Check sheet for the modelled part. Datum: model origin and axes. Units: mm. A direction names the side the tool comes from. Give positions to 0.01 mm unless a question says otherwise; leave off trailing zeros. Loops run counter-clockwise (first coordinate to the right, second up) from the corner with the lowest first, then second, coordinate; pieces in that order, holes last. Notation, with made-up numbers: (62.25, 86.5) - (105.25, 86.5) arc R10 ccw to (105.25, 94.5) - close; hole circle Ø7 at (-36.5, 26). An arc over 180 degrees is marked (long way). Use CSV: the item, a comma, the result in double quotes.
from build123d import *

# Parameters (mm, degrees)
SKETCH1_R               = 46.5
SKETCH1_R_2             = 36
BOSS_EXTRUDE1_DEPTH     = 2.325
BOSS_EXTRUDE2_START     = -2
SKETCH2_R               = 36
SKETCH2_R_2             = 33.63888889
BOSS_EXTRUDE2_DEPTH     = 2
CUT_EXTRUDE1_DEPTH      = 66.925127986
CUT_EXTRUDE1_DEPTH_BACK = 66.925127986
SKETCH3_R               = 1.25


with BuildPart() as part:
    # Sketch1 → Boss-Extrude1 (new, symmetric)
    with BuildSketch(Plane.XY):
        Circle(SKETCH1_R)
        Circle(SKETCH1_R_2, mode=Mode.SUBTRACT)
    extrude(amount=BOSS_EXTRUDE1_DEPTH, both=True)

    # Sketch2 → Boss-Extrude2 (add)
    with BuildSketch(Plane.XY.offset(2.325).offset(BOSS_EXTRUDE2_START)):
        Circle(SKETCH2_R)
        Circle(SKETCH2_R_2, mode=Mode.SUBTRACT)
    extrude(amount=BOSS_EXTRUDE2_DEPTH)

    # Sketch3 → Cut-Extrude1 (cut, two sides: drawn at the far end of the back side and taken through both)
    with BuildSketch(Plane.XY.offset(2.325).offset(-CUT_EXTRUDE1_DEPTH_BACK)):
        with Locations((-15.560126668, -38.202682603)):
            Circle(SKETCH3_R)
        with Locations((-32.576806282, -25.304430293)):
            Circle(SKETCH3_R)
        with Locations((-40.864556961, -5.625876321)):
            Circle(SKETCH3_R)
        with Locations((-38.202682603, 15.560126668)):
            Circle(SKETCH3_R)
        with Locations((-25.304430293, 32.576806282)):
            Circle(SKETCH3_R)
        with Locations((-5.625876321, 40.864556961)):
            Circle(SKETCH3_R)
        with Locations((15.560126668, 38.202682603)):
            Circle(SKETCH3_R)
        with Locations((32.576806282, 25.304430293)):
            Circle(SKETCH3_R)
        with Locations((40.864556961, 5.625876321)):
            Circle(SKETCH3_R)
        with Locations((38.202682603, -15.560126668)):
            Circle(SKETCH3_R)
        with Locations((25.304430293, -32.576806282)):
            Circle(SKETCH3_R)
        with Locations((5.625876321, -40.864556961)):
            Circle(SKETCH3_R)
    extrude(amount=CUT_EXTRUDE1_DEPTH + CUT_EXTRUDE1_DEPTH_BACK, mode=Mode.SUBTRACT)


solid = part.part
1. Scan lines: line 1 along Y through (x, z) = (14.5, -1.45); line 2 along Y through (x, z) = (16, 1.8); line 3 along X through (y, z) = (15.5, 0.6). Record each from-to range of solid material in increasing order.
Completed:
line 1,"y = -44.18 to -32.95, 32.95 to 37.54, 38.86 to 44.18"
line 2,"y = -43.66 to -29.59, 29.59 to 37.03, 39.37 to 43.66"
line 3,"x = -43.84 to -39.45, -36.95 to -29.86, 29.86 to 43.84"
2. Go/stop test with flat-tipped pins: pin 1 Ø3 at (x, y) = (25.3, -32.58) entering from -Z (3 decimals); pin 2 Ø1.5 at (x, y) = (-25.3, 32.58) entering from -Z; pin 3 Ø2 at (y, z) = (18, -1) entering from -X; pin 4 Ø2 at (y, z) = (29.5, -0.5) entering from -X. Record where each tip stops, or that it passes through.
Completed:
pin 1,"stops at z = -2.325"
pin 2,"passes through"
pin 3,"stops at x = -43.28"
pin 4,"stops at x = -36.74"
3. Set-up check for faces 5 (the face through (-39.124, 16.405, -0.033)), 6 (the face through (-30, 16, 0.325)): record each of +Z, -Z, +X, -X, +Y, -Y from which the full face is reachable in a straight line by a thin tool's end or side.
Completed:
face 5,"+Z, -Z"
face 6,"-Z"
4. Sectioned sample at C-C, the plane z = -0.5. State how many separate pieces and enclosed holes the cut face has, and give its area (3 significant figures).
Completed:
separate pieces,"1"
enclosed holes,"13"
area,"2,660 mm²"
5. Sectioned sample at A-A, the plane x = 0. Record the boundary of the cut face in (y, z) (3 decimals), and give its area (3 significant figures).
Completed:
outline,"(-46.5, -2.325) - (-36, -2.325) - (-36, 0.325) - (-33.639, 0.325) - (-33.639, 2.325) - (-46.5, 2.325) - close; (33.639, 0.325) - (36, 0.325) - (36, -2.325) - (46.5, -2.325) - (46.5, 2.325) - (33.639, 2.325) - close"
area,"107 mm²"
6. Release check for a two-part mould opening along Y. For faces 1 (the face through (-26.695, -20.469, 1.311)), 2 (the face through (24, 24, 2.325)), 3 (the face through (37.21, -16.32, -0.03)), 4 (the face through (44.35, 13.97, 0.03)) record: released by +Y, released by -Y, zero draft, split by the parting line, or undercut.
Completed:
face 1,"undercut"
face 2,"zero draft"
face 3,"undercut"
face 4,"split by the parting line"
